Study the drawing (mm; zero at the part's minimum x, y, z) and answer. Coordinates: 2 decimals unless noted, no trailing zeros. Loops run counter-clockwise (first coordinate to the right, second up) from the corner with the lowest first, then second, coordinate; pieces in that order, holes last. Notation, with made-up numbers: (-24, 1) -> (-7, 1) arc R22 cw to (-7, 23) -> close; hole circle Ø1 at (73, 27). An arc over 180 degrees is marked (long way). One line per question, with ' | ' between items.
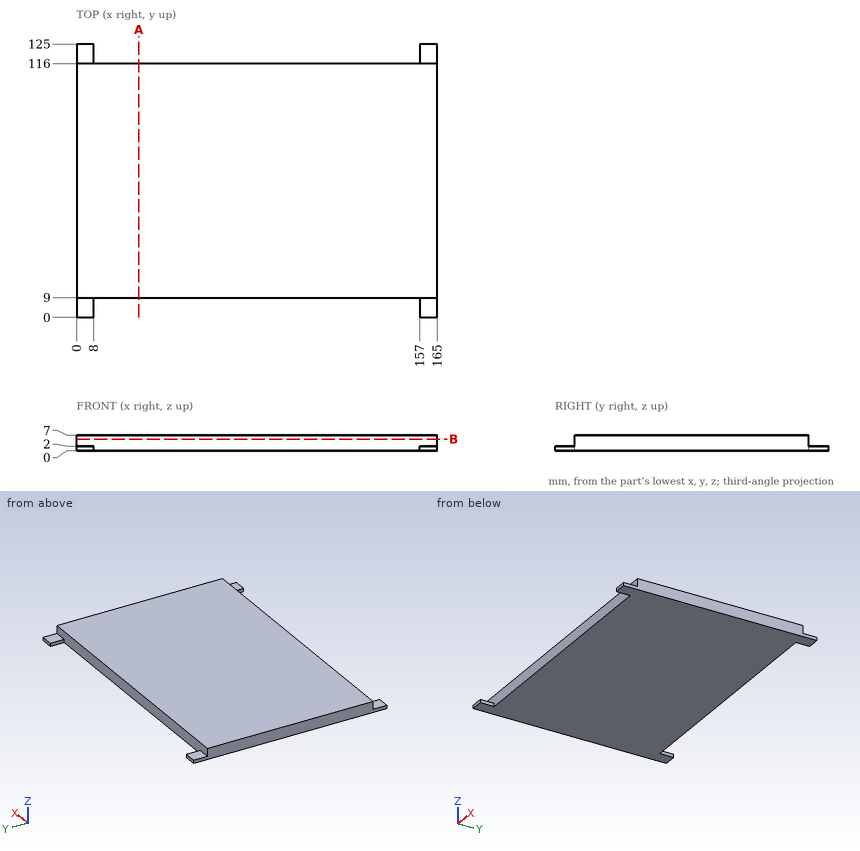
1) Flat-ended cylindrical pins translate along their axes: pin 1 (2 mm diameter, centred on x = 98.5, z = 2.5, fed in from +Y); pin 2 (4 mm diameter, centred on x = 3, y = 6, fed in from +Z); pin 3 (2 mm diameter, centred on x = 48, z = 4.5, fed in from -Y). Find the tip coordinate at first contact, or state that the pin passes through.
Check values:
pin 1: stops at y = 116 | pin 2: stops at z = 2 | pin 3: stops at y = 9
2) Find the intervals of material crossed by line 1 along Y through (x, z) = (103, 3.5), in increasing order.
Check values:
line 1: y = 9 to 116
3) Find section B-B (z = 5.25). Write down the section's boundary in (x, y), plus the area to 3 significant figures.
Check values:
outline: (0, 9) -> (165, 9) -> (165, 116) -> (0, 116) -> close | area: 17,700 mm^2
4) Find section A-A (x = 28.5). Write down the section's boundary in (y, z).
Check values:
outline: (9, 0) -> (116, 0) -> (116, 7) -> (9, 7) -> close
